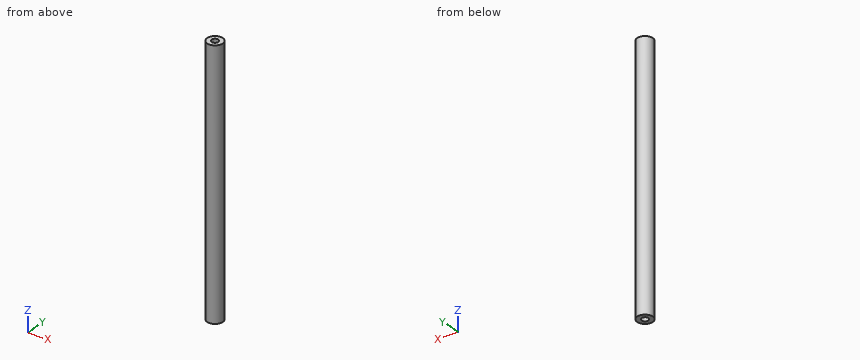
Autodesk Inventor part; units mm, degrees
ref_plane "YZ Plane" through (0, 0, 0) normal (1, 0, 0) x (0, 1, 0)
ref_plane "XZ Plane" through (0, 0, 0) normal (0, 1, 0) x (-1, 0, 0)
ref_plane "XY Plane" through (0, 0, 0) normal (0, 0, 1) x (1, 0, 0)
sketch "スケッチ1" plane through (0, 0, 0) normal (0, 0, 1) x (1, 0, 0)
  circle A0 centre (0, 0) radius 4
  circle A1 centre (0, 0) radius 1.75
  dimension "d0" = 8
  dimension "d1" = 3.5
extrude "押し出し1" add sketch "スケッチ1" along normal blind 132.2 contours A0 | A1
extrude "押し出し2" cut sketch "スケッチ1" along normal blind 10 contours A1
sketch "スケッチ2" plane through (0, 0, 132.2) normal (0, 0, 1) x (1, 0, 0)
  circle A0 centre (0, 0) radius 1.75
  dimension "d6" = 3.5
extrude "押し出し3" cut sketch "スケッチ2" against normal blind 10
equation "\"d6\" = d1"
properties part number "棒" material "アルミニウム 2014-T4"
The listing builds one solid part. Answer for the finished solid, in the listing's coordinates (mm). Give positions to 0.01 mm unless a question says otherwise; leave off trailing zeros. Write each loop counter-clockwise with the first axis right and the second up, starting at its lowest first coordinate (ties: lowest second). Pieces come first, ordered by that corner, then holes. Notation, with made-up numbers: (-24, 80) -> (-17, 80) arc R28 ccw to (-17, 119) -> close; hole circle Ø9 at (-6, 82). An arc over 180 degrees is marked (long way). Write item = value, one per line. Start each with the question number.
1) The part is cut by section C-C, the plane z = 14.5. Determine the outline of the cut face in (x, y), and give its area (3 significant figures).
2) Each of these flat-tipped pins is pushed along its axis until it touches: pin 1 (3 mm diameter, centred on x = 0, y = 0, fed in from -Z); pin 2 (4 mm diameter, centred on y = 3, z = 93, fed in from -X); pin 3 (3 mm diameter, centred on x = 0, y = 0, fed in from +Z). Where does it stop, or does it pass through?
3) Straight lines are drawn through the part: line 1 along Y through (x, z) = (0, 7.5); line 2 along Z through (x, y) = (1, 0.75); line 3 along X through (y, z) = (0.25, 60). For each, find the intervals that lie inside material, in ascending order.
4) The part is cut by section A-A, the plane x = 0. Determine the outline of the cut face in (y, z).
Solutions:
q1.outline = circle Ø8 at (0, 0)
q1.area = 50.3 mm²
q2.pin_1 = 10
q2.pin_2 = -3.87
q2.pin_3 = 122.2
q3.line_1 = -4 to -1.75, 1.75 to 4
q3.line_2 = 10 to 122.2
q3.line_3 = -3.99 to 3.99
q4.outline = (-4, 0) -> (-1.75, 0) -> (-1.75, 10) -> (1.75, 10) -> (1.75, 0) -> (4, 0) -> (4, 132.2) -> (1.75, 132.2) -> (1.75, 122.2) -> (-1.75, 122.2) -> (-1.75, 132.2) -> (-4, 132.2) -> close
